from build123d import *

# Parameters (mm, degrees)
EXTRUDE_355_DEPTH      = 50
SKETCH_2_W             = 90
SKETCH_2_H             = 90
CUT_EXTRUDE_705_DEPTH  = 45
SKETCH_3_R             = 3.5
SKETCH_3_R_2           = 1.5
TYPE_C_DEPTH           = 4
TYPE_C_START           = -2
SKETCH_3_2_R           = 1.5
TYPE_C_2_DEPTH         = 2
SKETCH_4_W             = 36.625
SKETCH_4_H             = 10
TYPE_C_3_DEPTH         = 3
SKETCH_5_W             = 10
SKETCH_5_H             = 5
TYPE_C_4_DEPTH         = 2
SKETCH_6_R             = 3
SKETCH_6_R_2           = 1.5
EXTRUDE_2034_DEPTH     = 5
SKETCH_7_W             = 30
SKETCH_7_H             = 20
OLED_DEPTH             = 5
SKETCH_8_W             = 44
SKETCH_8_H             = 34
OLED_2_DEPTH           = 2
SKETCH_9_R             = 4
SKETCH_9_R_2           = 2
CUT_EXTRUDE_2931_DEPTH = 2.5
SKETCH_9_2_R           = 2
CUT_EXTRUDE_2975_DEPTH = 5
SKETCH_10_W            = 84
SKETCH_10_H            = 40
CUT_EXTRUDE_9_DEPTH    = 5
SKETCH_11_W            = 23.6875
SKETCH_11_H            = 3
CUT_EXTRUDE_10_DEPTH   = 2
SKETCH_12_W            = 84
SKETCH_12_H            = 3
CUT_EXTRUDE_11_DEPTH   = 3
SKETCH_14_W            = 10
SKETCH_14_H            = 3
EXTRUDE_1_DEPTH        = 25
SKETCH_14_2_W          = 10
SKETCH_14_2_H          = 3
CUT_EXTRUDE_12_DEPTH   = 10


with BuildPart() as part:
    # 草图1 → Extrude 355 (new body)
    with BuildSketch(Plane(origin=(0, 0, 0), x_dir=(1, 0, 0), z_dir=(0, 1, 0))):
        with BuildLine():
            Line((3, 0), (97, 0))
            ThreePointArc((97, 0), (99.121320344, 0.878679656), (100, 3))
            Line((100, 3), (100, 97))
            ThreePointArc((100, 97), (99.121320344, 99.121320344), (97, 100))
            Line((97, 100), (3, 100))
            ThreePointArc((3, 100), (0.878679656, 99.121320344), (0, 97))
            Line((0, 97), (0, 3))
            ThreePointArc((0, 3), (0.878679656, 0.878679656), (3, 0))
        make_face()
    extrude(amount=EXTRUDE_355_DEPTH)

    # 草图2 → Cut-Extrude 705 (cut)
    with BuildSketch(Plane(origin=(0, 50, 0), x_dir=(1, 0, 0), z_dir=(0, 1, 0))):
        with Locations((50, 50)):
            Rectangle(SKETCH_2_W, SKETCH_2_H)
    extrude(amount=-CUT_EXTRUDE_705_DEPTH, mode=Mode.SUBTRACT)

    # 草图3 → TYPE-C (add)
    # profile 1 of 2: a face of its own
    with BuildSketch(Plane(origin=(0, 5, 0), x_dir=(1, 0, 0), z_dir=(0, 1, 0))):
        with Locations(Location((37.1875, 86, 0), (0, 0, 90))):
            Circle(SKETCH_3_R)
        with Locations(Location((37.1875, 86, 0), (0, 0, 270))):
            Circle(SKETCH_3_R_2, mode=Mode.SUBTRACT)
    # profile 2 of 2: a face of its own
    with BuildSketch(Plane(origin=(0, 5, 0), x_dir=(1, 0, 0), z_dir=(0, 1, 0))):
        with Locations(Location((62.8125, 86, 0), (0, 0, 90))):
            Circle(SKETCH_3_R)
        with Locations(Location((62.8125, 86, 0), (0, 0, 270))):
            Circle(SKETCH_3_R_2, mode=Mode.SUBTRACT)
    extrude(amount=TYPE_C_DEPTH)

    # 草图3<2> → TYPE-C 2 (cut)
    with BuildSketch(Plane(origin=(0, 5, 0), x_dir=(1, 0, 0), z_dir=(0, 1, 0)).offset(TYPE_C_START)):
        with Locations(Location((37.1875, 86, 0), (0, 0, 270))):
            Circle(SKETCH_3_2_R)
        with Locations(Location((62.8125, 86, 0), (0, 0, 270))):
            Circle(SKETCH_3_2_R)
    extrude(amount=TYPE_C_2_DEPTH, mode=Mode.SUBTRACT)

    # 草图4 → TYPE-C 3 (cut)
    with BuildSketch(Plane.XY.offset(-95)):
        with Locations((50, 13)):
            Rectangle(SKETCH_4_W, SKETCH_4_H)
    extrude(amount=-TYPE_C_3_DEPTH, mode=Mode.SUBTRACT)

    # 草图5 → TYPE-C 4 (cut)
    with BuildSketch(Plane.XY.offset(-98)):
        with Locations((50, 12.5)):
            Rectangle(SKETCH_5_W, SKETCH_5_H)
    extrude(amount=-TYPE_C_4_DEPTH, mode=Mode.SUBTRACT)

    # 草图6 → Extrude 2034 (add)
    # profile 1 of 4: a face of its own
    with BuildSketch(Plane(origin=(0, 0, -5), x_dir=(-1, 0, 0), z_dir=(0, 0, -1))):
        with Locations(Location((-87, 44.5, 0), (0, 0, 180))):
            Circle(SKETCH_6_R)
        with Locations((-87, 44.5)):
            Circle(SKETCH_6_R_2, mode=Mode.SUBTRACT)
    # profile 2 of 4: a face of its own
    with BuildSketch(Plane(origin=(0, 0, -5), x_dir=(-1, 0, 0), z_dir=(0, 0, -1))):
        with Locations(Location((-87, 24.5, 0), (0, 0, 180))):
            Circle(SKETCH_6_R)
        with Locations((-87, 24.5)):
            Circle(SKETCH_6_R_2, mode=Mode.SUBTRACT)
    # profile 3 of 4: a face of its own
    with BuildSketch(Plane(origin=(0, 0, -5), x_dir=(-1, 0, 0), z_dir=(0, 0, -1))):
        with Locations(Location((-13, 44.5, 0), (0, 0, 180))):
            Circle(SKETCH_6_R)
        with Locations((-13, 44.5)):
            Circle(SKETCH_6_R_2, mode=Mode.SUBTRACT)
    # profile 4 of 4: a face of its own
    with BuildSketch(Plane(origin=(0, 0, -5), x_dir=(-1, 0, 0), z_dir=(0, 0, -1))):
        with Locations(Location((-13, 10.5, 0), (0, 0, 180))):
            Circle(SKETCH_6_R)
        with Locations((-13, 10.5)):
            Circle(SKETCH_6_R_2, mode=Mode.SUBTRACT)
    extrude(amount=EXTRUDE_2034_DEPTH)

    # 草图7 → OLED (cut)
    with BuildSketch(Plane.XY):
        with Locations((50, 30)):
            Rectangle(SKETCH_7_W, SKETCH_7_H)
    extrude(amount=-OLED_DEPTH, mode=Mode.SUBTRACT)

    # 草图8 → OLED 2 (cut)
    with BuildSketch(Plane(origin=(0, 0, -5), x_dir=(-1, 0, 0), z_dir=(0, 0, -1))):
        with Locations((-50, 30)):
            Rectangle(SKETCH_8_W, SKETCH_8_H)
    extrude(amount=-OLED_2_DEPTH, mode=Mode.SUBTRACT)

    # 草图9 → Cut-Extrude 2931 (cut)
    # profile 1 of 2: a face of its own
    with BuildSketch(Plane.XZ):
        with Locations(Location((80, -50, 0), (0, 0, 270))):
            Circle(SKETCH_9_R)
        with Locations(Location((80, -50, 0), (0, 0, 270))):
            Circle(SKETCH_9_R_2, mode=Mode.SUBTRACT)
    # profile 2 of 2: a face of its own
    with BuildSketch(Plane.XZ):
        with Locations(Location((20, -50, 0), (0, 0, 270))):
            Circle(SKETCH_9_R)
        with Locations(Location((20, -50, 0), (0, 0, 270))):
            Circle(SKETCH_9_R_2, mode=Mode.SUBTRACT)
    extrude(amount=-CUT_EXTRUDE_2931_DEPTH, mode=Mode.SUBTRACT)

    # 草图9<2> → Cut-Extrude 2975 (cut)
    with BuildSketch(Plane.XZ):
        with Locations(Location((80, -50, 0), (0, 0, 270))):
            Circle(SKETCH_9_2_R)
        with Locations(Location((20, -50, 0), (0, 0, 270))):
            Circle(SKETCH_9_2_R)
    extrude(amount=-CUT_EXTRUDE_2975_DEPTH, mode=Mode.SUBTRACT)

    # 草图10 → 切除-拉伸9 (cut)
    with BuildSketch(Plane(origin=(0, 0, -100), x_dir=(-1, 0, 0), z_dir=(0, 0, -1))):
        with Locations((-50, 30)):
            Rectangle(SKETCH_10_W, SKETCH_10_H)
    extrude(amount=-CUT_EXTRUDE_9_DEPTH, mode=Mode.SUBTRACT)

    # 草图11 → 切除-拉伸10 (cut)
    with BuildSketch(Plane(origin=(0, 10, 0), x_dir=(1, 0, 0), z_dir=(0, 1, 0))):
        with Locations((80.15625, 96.5)):
            Rectangle(SKETCH_11_W, SKETCH_11_H)
        with Locations((19.84375, 96.5)):
            Rectangle(SKETCH_11_W, SKETCH_11_H)
    extrude(amount=-CUT_EXTRUDE_10_DEPTH, mode=Mode.SUBTRACT)

    # 草图12 → 切除-拉伸11 (cut)
    with BuildSketch(Plane(origin=(0, 8, 0), x_dir=(1, 0, 0), z_dir=(0, 1, 0))):
        with Locations((50, 96.5)):
            Rectangle(SKETCH_12_W, SKETCH_12_H)
    extrude(amount=-CUT_EXTRUDE_11_DEPTH, mode=Mode.SUBTRACT)

    # 草图14 → 凸台-拉伸1 (add)
    with BuildSketch(Plane(origin=(0, 50, 0), x_dir=(1, 0, 0), z_dir=(0, 1, 0))):
        with Locations((13, 96.5)):
            Rectangle(SKETCH_14_W, SKETCH_14_H)
        with Locations((87, 96.5)):
            Rectangle(SKETCH_14_W, SKETCH_14_H)
    extrude(amount=-EXTRUDE_1_DEPTH)

    # 草图14<2> → 切除-拉伸12 (cut)
    with BuildSketch(Plane(origin=(0, 50, 0), x_dir=(1, 0, 0), z_dir=(0, 1, 0))):
        with Locations((13, 96.5)):
            Rectangle(SKETCH_14_2_W, SKETCH_14_2_H)
        with Locations((87, 96.5)):
            Rectangle(SKETCH_14_2_W, SKETCH_14_2_H)
    extrude(amount=-CUT_EXTRUDE_12_DEPTH, mode=Mode.SUBTRACT)


solid = part.part
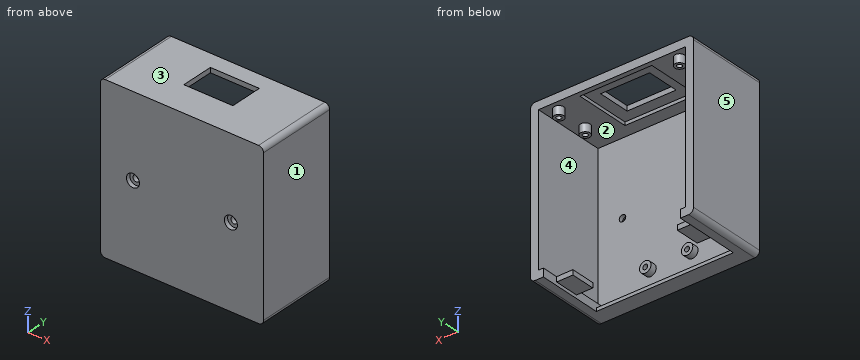
Model file for the job. Use its own axes, mm. Face numbers are marked on the shaded views. A direction names the side the tool comes from. Round coordinates to 2 decimals unless told otherwise and drop trailing zeros. Order: outer loops, then holes, each group sorted by start corner. A loop starts at its lowest first (then second) coordinate and runs counter-clockwise, first axis right, second up. Notation, with made-up numbers: M 36,59.25 L 81,59.25 A11 ccw 81,71.25 Z; hole C 39,58.5 d9. An arc over 180 degrees is marked long. Write each question's results on one line, items separated by ' | '. Start each with the question number.
(1) Saw through at B-B, the plane x = 80. Give the cut face in (y, z).
(2) Drop flat-ended pins along their axis: pin 1 (3.5 mm diameter, centred on x = 36.5, z = -85.5, fed in from +Y); pin 2 (2 mm diameter, centred on x = 61.5, y = 38.5, fed in from -Z); pin 3 (6.5 mm diameter, centred on x = 13, y = 45.5, fed in from -Z); pin 4 (12 mm diameter, centred on x = 43, y = 17, fed in from -Z). Give the stop position or say it passes through.
(3) Which spindle directions (+Z, -Z, +X, -X, +Y, -Y) get a long thin tool onto all of the face, cutting with end or side? Do the marked faces 1 and 2. Say none if no direction does.
(4) Saw through at A-A, the plane z = -8. State how many separate pieces and enclosed holes the cut face has, then the cut area to 3 significant figures.
(5) Probe probe 1 along X at (y, z) = (4.55, -86); probe 2 along X at (y, z) = (1, -50); probe 3 along X at (y, z) = (13, -11). List the from-to ranges inside material, lowest first. Write a range as from..to.
(6) Saw through at D-D, the plane z = -28. Give the cut face in (x, y).
(7) Saw through at C-C, the plane y = 32. Give the cut face in (x, z).
(8) Two-plate mould, pull along Z, no slides. Class the marked faces 3, 4 and 5: pulls with the +Z half, pulls with the -Z half, needs draft (parallel to the pull), parting line crosses it, or undercut.
Established:
1) outline: M 0,-100 L 10,-100 L 10,-98 L 5,-98 L 5,-52 L 2.5,-52 L 2.5,-54 L 0,-54 Z; M 0,-46 L 2.5,-46 L 2.5,-48 L 5,-48 L 5,-5 L 50,-5 L 50,0 L 0,0 Z
2) pin 1: stops at y = 9 | pin 2: passes through | pin 3: stops at z = -10 | pin 4: stops at z = -5
3) face 1: +Z, -Z, +X, +Y, -Y | face 2: none
4) separate pieces: 5 | enclosed holes: 4 | area: 1,030 mm^2
5) probe 1: x = 0..35.69, 38.69..61.31, 64.31..100 | probe 2: x = 0..16, 24..76, 84..100 | probe 3: x = 0..5, 95..100
6) outline: M 0,0 L 100,0 L 100,50 L 95,50 L 95,5 L 5,5 L 5,50 L 0,50 Z
7) outline: M 0,-97 A3 ccw 3,-100 L 8,-100 L 8,-98 L 18,-98 L 18,-95 L 5,-95 L 5,-5 L 28,-5 L 28,-3 L 35,-3 L 35,0 L 3,0 A3 ccw 0,-3 Z; M 65,-3 L 72,-3 L 72,-5 L 95,-5 L 95,-95 L 82,-95 L 82,-98 L 92,-98 L 92,-100 L 97,-100 A3 ccw 100,-97 L 100,-3 A3 ccw 97,0 L 65,0 Z
8) face 3: pulls with the +Z half | face 4: undercut | face 5: needs draft
